The listing builds one solid part. Answer for the finished solid, in the listing's coordinates (mm). A direction names the side the tool comes from. Round coordinates to 2 decimals unless told otherwise and drop trailing zeros. Order: outer loops, then holes, each group sorted by start corner. A loop starts at its lowest first (then second) coordinate and runs counter-clockwise, first axis right, second up. Notation, with made-up numbers: M 71,78.5 L 118,78.5 A22 ccw 118,117.5 Z; hole C -24.5,9 d10. An arc over 180 degrees is marked long. Write item = value, one per line. Start each with the question number.
(1) Straight lines are drawn through the part: probe 1 along Z at (x, y) = (3.25, -3); probe 2 along Z at (x, y) = (-1.5, -0.75); probe 3 along X at (y, z) = (0.25, 21.5). For each, find the intervals that lie inside material, in ascending order. Write a range as from..to.
(2) Each of these flat-tipped pins is pushed along its axis until it touches: pin 1 (1.5 mm diameter, centred on y = 2, z = 87, fed in from -X); pin 2 (1.5 mm diameter, centred on y = -5, z = 18, fed in from +X); pin 3 (5 mm diameter, centred on y = -2.5, z = 35, fed in from +X); pin 4 (1 mm diameter, centred on x = -0.5, y = -1, fed in from +Z). Where does it stop, or does it pass through?
(3) A cutting plane is placed at A-A, the plane y = 0. Determine the outline of the cut face in (x, z), and give its area (3 significant figures).
(4) For a pull along Y with two mould halves and no side action, classify faces 1 (the face through (3, 3, 140)), 2 (the face through (3, 0, 146)), 3 (the face through (-0.867, 3.905, 69.426)) as released by +Y, released by -Y, zero draft, split by the parting line, or undercut.
(5) Which of the six approach directions +Z, -Z, +X, -X, +Y, -Y give full straight-line access (tool end or side, diameter ignored) to faces 4 (the face through (0, 0, 0)), 5 (the face through (0, 0, 144))?
(6) A cutting plane is placed at B-B, the plane z = 25. Determine the outline of the cut face in (x, y), and give its area (3 significant figures).
Autodesk Inventor part; units mm, degrees
ref_plane "YZ Plane" through (0, 0, 0) normal (1, 0, 0) x (0, 1, 0)
ref_plane "XZ Plane" through (0, 0, 0) normal (0, 1, 0) x (-1, 0, 0)
ref_plane "XY Plane" through (0, 0, 0) normal (0, 0, 1) x (1, 0, 0)
sketch "Sketch1" plane through (0, 0, 0) normal (0, 0, 1) x (1, 0, 0)
  circle A0 centre (0, 0) radius 4
  dimension "Diameter" = 8
extrude "Extrusion1" add sketch "Sketch1" along normal blind 140
sketch "Sketch2" plane through (0, 0, 140) normal (0, 0, 1) x (1, 0, 0)
  circle A0 centre (0, 0) radius 4
  circle A1 centre (0, 0) radius 6.5
  dimension "Head_Diameter" = 13
extrude "Extrusion2" add sketch "Sketch2" along normal blind 8 contours A0 | A1
sketch "Sketch3" plane through (0, 0, 148) normal (0, 0, 1) x (1, 0, 0)
  circle A0 centre (0, 0) radius 6.5
  circle A1 centre (0, 0) radius 3.4641 construction
  line L0 (0, 3.4641) -> (3, 1.7321)
  line L1 (3, -1.7321) -> (3, 1.7321)
  line L2 (0, 3.4641) -> (-3, 1.7321)
  line L3 (-3, -1.7321) -> (-3, 1.7321)
  line L4 (-3, -1.7321) -> (0, -3.4641)
  line L5 (3, -1.7321) -> (0, -3.4641)
  dimension "Hex_Width" = 6
extrude "Extrusion3" cut sketch "Sketch3" against normal blind 4 contours L0 L1 L5 L4 L3 L2
thread "Thread1"
chamfer "Chamfer1" distance 0.8 angle 45 2 edges at (-6.5, 0, 148) (-4, 0, 0)
equation "\"d9\" = ThreadLength"
equation "\"d12\" = Chamfer"
equation "\"ThreadLength\" = 28"
properties part number "SCREW, SOCKET HD, P, 12.9, M8X1.25X140MM" material "Steel, Mild"
Reported:
q1.probe_1 = 140..148
q1.probe_2 = 0..144
q1.probe_3 = -3.99..3.99
q2.pin_1 = -3.8
q2.pin_2 = through
q2.pin_3 = 4
q2.pin_4 = 144
q3.outline = M -6.5,140 L -4,140 L -4,0.8 L -3.2,0 L 3.2,0 L 4,0.8 L 4,140 L 6.5,140 L 6.5,147.2 L 5.7,148 L 3,148 L 3,144 L -3,144 L -3,148 L -5.7,148 L -6.5,147.2 Z
q3.area = 1,200 mm²
q4.face_1 = zero draft
q4.face_2 = undercut
q4.face_3 = split by the parting line
q5.face_4 = -Z, +X, -X, +Y, -Y
q5.face_5 = +Z
q6.outline = C 0,0 d8
q6.area = 50.3 mm²
